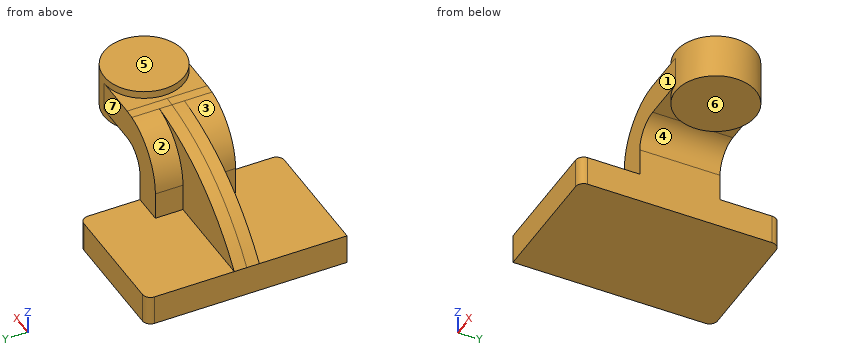
from build123d import *

# Parameters (mm, degrees)
F1_DEPTH = 63.5
F2_DEPTH = 25.4
F0_W     = 25.4
F0_H     = 19.05
F3_DEPTH = 25.4
F4_DEPTH = 7.9375
F6_R     = 5.08


with BuildPart() as f1:
    # F0 (on Front) → F1 (new body, symmetric)
    with BuildSketch(Plane.XZ):
        Polygon((41.275, -9.525), (41.275, 9.525), (22.225, 9.525), (-41.275, 9.525), (-41.275, -9.525), align=None)
    extrude(amount=F1_DEPTH, both=True)

    # F0 (on Front) → F2 (join, symmetric)
    with BuildSketch(Plane.XZ):
        with BuildLine():
            Line((22.225, 9.525), (41.275, 9.525))
            Line((41.275, 9.525), (41.275, 27.0002))
            ThreePointArc((41.275, 27.0002), (45.9246798487, 38.2255201513), (57.15, 42.8752))
            Line((57.15, 42.8752), (60.325, 42.8752))
            Line((60.325, 42.8752), (60.325, 61.9252))
            Line((60.325, 61.9252), (57.15, 61.9252))
            add(Edge.make_bspline(
                [(51.3437067014, 61.4391689615), (53.2701840595, 61.6380826353), (55.2059301459, 61.8000229845), (57.15, 61.9252)],
                knots=[105.8784898715, 105.8784898715, 105.8784898715, 105.8784898715, 111.5045361635, 111.5045361635, 111.5045361635, 111.5045361635], degree=3))
            ThreePointArc((51.3437067014, 61.4391689615), (30.4803504105, 49.5498211891), (22.225, 27.0002))
            Line((22.225, 27.0002), (22.225, 9.525))
        make_face()
    extrude(amount=F2_DEPTH, both=True)

    # F0 (on Front) → F3 (join, symmetric)
    with BuildSketch(Plane.XZ):
        with Locations((73.025, 52.4002)):
            Rectangle(F0_W, F0_H)
    extrude(amount=F3_DEPTH, both=True)

    # F0 (on Front) → F4 (join, symmetric)
    with BuildSketch(Plane.XZ):
        with BuildLine():
            Line((-41.275, 9.525), (22.225, 9.525))
            Line((22.225, 9.525), (22.225, 27.0002))
            ThreePointArc((22.225, 27.0002), (30.4803504105, 49.5498211891), (51.3437067014, 61.4391689615))
            add(Edge.make_bspline(
                [(-41.275, 9.525), (-17.8836826393, 40.8575650231), (15.0886702409, 57.6957444853), (51.3437067014, 61.4391689615)],
                knots=[0, 0, 0, 0, 105.8784898715, 105.8784898715, 105.8784898715, 105.8784898715], degree=3))
        make_face()
    extrude(amount=F4_DEPTH, both=True)

    # F0 (on Front) → F5 (revolve)
    with BuildSketch(Plane.XZ):
        Polygon((85.725, 61.9252), (85.725, 42.8752), (85.725, 38.1), (111.125, 38.1), (111.125, 66.675), (85.725, 66.675), align=None)
    revolve(axis=Axis((85.725, 0, 52.3875), (0, 0, 1)))

    # F6
    f6_edges = [f1.edges().sort_by_distance(p)[0] for p in [
        (41.275, -63.5, 0),
        (-41.275, 63.5, 0),
        (41.275, 63.5, 0),
    ]]
    fillet(f6_edges, radius=F6_R)


solid = f1.part
The listing builds one solid part. Answer for the finished solid, in the listing's coordinates (mm). Face numbers are marked on the shaded views. A direction names the side the tool comes from. Round coordinates to 2 decimals unless told otherwise and drop trailing zeros. Write each loop counter-clockwise with the first axis right and the second up, starting at its lowest first coordinate (ties: lowest second). Pieces come first, ordered by that corner, then holes. Notation, with made-up numbers: M 87.5,-38 L 113.5,-38 A21 cw 113.5,-34 Z; hole C -29,85.5 d3. An arc over 180 degrees is marked long. Write each question's results on one line, items separated by ' | '. Start each with the question number.
Item 1: Which of the six approach directions +Z, -Z, +X, -X, +Y, -Y give full straight-line access (tool end or side, diameter ignored) to the marked faces 1, 2, 3 and 4?
Item 2: Straight lines are drawn through the part: probe 1 along X at (y, z) = (43, 8.5) (3 decimals); probe 2 along Y at (x, z) = (86.5, 52.5); probe 3 along Z at (x, y) = (59.5, -4). For each, find the intervals that lie inside material, in ascending order.
Item 3: Find section B-B on y = 29. Write down the section's boundary in (x, z) (3 decimals), and give its area (3 significant figures).
Item 4: Given pin 1 Ø23 at (x, y) = (70, 3.5) entering from -Z; pin 2 Ø12 at (x, y) = (2.5, 17.5) entering from +Z (3 decimals); pin 3 Ø5 at (y, z) = (-15, 16) entering from -X (3 decimals), each flat-ended and moving along its own axis, determine where each tip first touches the part or whether it passes through.
Item 5: Find section A-A on z = -3.5. Write down the section's boundary in (x, y) (3 decimals).
Item 6: The mould has two halves that part along Z. Classify the marked faces 5, 6 and 7: +Z half, -Z half, draft (parallel to the pull), parting line (faces both ways), or undercut.
Answer block:
1) face 1: +Z, +X, -X, -Y | face 2: +Z, -X, +Y | face 3: +Z, -X, -Y | face 4: -Z, +Y, -Y
2) probe 1: x = -41.275 to 41.275 | probe 2: y = -25.39 to 25.39 | probe 3: z = 42.88 to 61.93
3) outline: M -41.275,-9.525 L 41.275,-9.525 L 41.275,9.525 L -41.275,9.525 Z | area: 1,570 mm²
4) pin 1: stops at z = 38.1 | pin 2: stops at z = 9.525 | pin 3: stops at x = 22.225
5) outline: M -41.275,-63.5 L 36.195,-63.5 A5.08 ccw 41.275,-58.42 L 41.275,58.42 A5.08 ccw 36.195,63.5 L -36.195,63.5 A5.08 ccw -41.275,58.42 Z
6) face 5: +Z half | face 6: -Z half | face 7: draft
